Check sheet for the modelled part. Datum: model origin and axes. Units: mm. Coordinates: 2 decimals unless noted, no trailing zeros. Write each loop counter-clockwise with the first axis right and the second up, starting at its lowest first coordinate (ties: lowest second). Pieces come first, ordered by that corner, then holes. Notation, with made-up numbers: (-27.5, -1.75) -> (5.5, -1.75) arc R12 ccw to (5.5, 13.25) -> close; hole circle Ø4 at (51.5, 60). An arc over 180 degrees is marked (long way). Put each result on its own line as item: value.
```python
from build123d import *

# Parameters (mm, degrees)
SALIENTE_EXTRUIR1_DEPTH = 6.2
CROQUIS2_R              = 3.175
CORTAR_EXTRUIR1_DEPTH   = 145.106369341


with BuildPart() as part:
    # Croquis1 → Saliente-Extruir1 (new body)
    with BuildSketch(Plane(origin=(0, 0, 0), x_dir=(1, 0, 0), z_dir=(0, 1, 0))):
        with BuildLine():
            Line((0, 0), (0, -79.550020016))
            Line((0, -79.550020016), (120, -79.550020016))
            Line((120, -79.550020016), (120, 0))
            Line((120, 0), (110, 0))
            ThreePointArc((110, 0), (60, -17.550020016), (10, 0))
            Line((10, 0), (0, 0))
        make_face()
    extrude(amount=SALIENTE_EXTRUIR1_DEPTH)

    # Croquis2 → Cortar-Extruir1 (cut, through all)
    with BuildSketch(Plane(origin=(0, 6.2, 0), x_dir=(1, 0, 0), z_dir=(0, 1, 0))):
        with Locations(Location((85, -39.775010008, 0), (0, 0, 270))):
            Circle(CROQUIS2_R)
    extrude(amount=-CORTAR_EXTRUIR1_DEPTH, mode=Mode.SUBTRACT)


solid = part.part
```
Q1. Cross-section at B-B (z = 5.5). Record the cut outline in (x, y), plus the area to 3 significant figures.
Recorded:
outline: (0, 0) -> (17.78, 0) -> (17.78, 6.2) -> (0, 6.2) -> close; (102.22, 0) -> (120, 0) -> (120, 6.2) -> (102.22, 6.2) -> close
area: 220 mm2
Q2. Cross-section at D-D (x = 105.5). Record the cut outline in (y, z), plus the area to 3 significant figures.
Recorded:
outline: (0, 3.35) -> (6.2, 3.35) -> (6.2, 79.55) -> (0, 79.55) -> close
area: 472 mm2
Q3. Depth check by flat-ended pin: P1, Ø2, axis at y = 2, z = 33, coming from the -X side; P2, Ø4, axis at x = 85, z = 39.78, coming from the +Y side; P3, Ø1.5, axis at x = 65.5, y = 1, coming from the -Z side. Enter the tip coordinate at first touch or a pass-through.
Recorded:
P1: stops at x = 0
P2: passes through
P3: stops at z = 17.31
Q4. Mould release check, pull along X, two halves, no side actions. Record for faces 1 (the cylindrical face through (87.68, 3.14, 41.48)), 2 (the flat face through (59, 3, 79.55)), 3 (the flat face through (0, 3, 39)): released by +X, released by -X, zero draft, split by the parting line, or undercut.
Recorded:
face 1: undercut
face 2: zero draft
face 3: released by -X
Q5. Cross-section at A-A (y = 4.75). Record the cut outline in (x, z) (3 decimals), plus the area to 3 significant figures.
Recorded:
outline: (0, 0) -> (10, 0) arc R80 cw to (110, 0) -> (120, 0) -> (120, 79.55) -> (0, 79.55) -> close; hole circle Ø6.35 at (85, 39.775)
area: 8,320 mm2
Q6. Material ranges on line 1 along X through (y, z) = (2.5, 40); line 2 along X through (y, z) = (1.25, 11.5); line 3 along Z through (x, y) = (80, 4), recorded low to high.
Recorded:
line 1: x = 0 to 81.83, 88.17 to 120
line 2: x = 0 to 29.48, 90.52 to 120
line 3: z = 15.01 to 79.55
Q7. Cross-section at C-C (x = 85). Record the cut outline in (y, z), plus the area to 3 significant figures.
Recorded:
outline: (0, 13.54) -> (6.2, 13.54) -> (6.2, 36.6) -> (0, 36.6) -> close; (0, 42.95) -> (6.2, 42.95) -> (6.2, 79.55) -> (0, 79.55) -> close
area: 370 mm2
